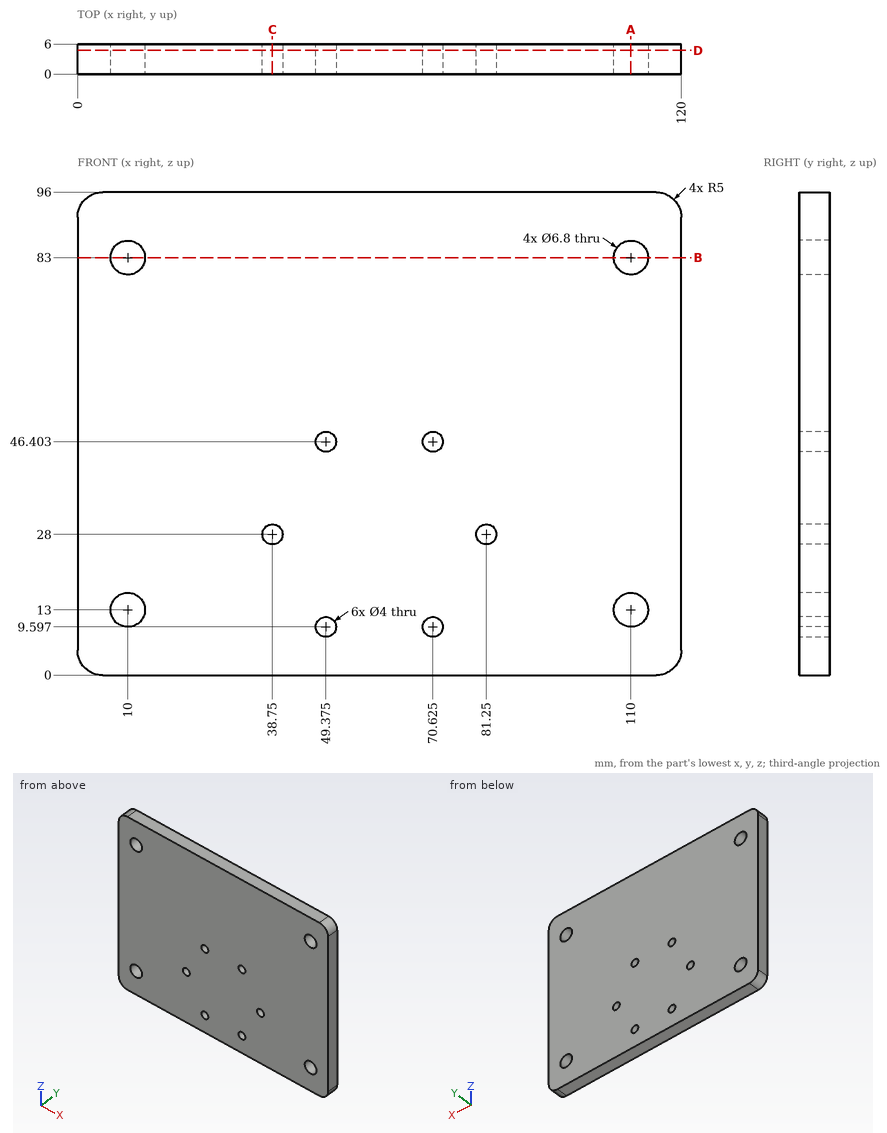
Part print with two shaded views. Sizes in mm from the minimum x, y, z corner. Round coordinates to 2 decimals unless told otherwise and drop trailing zeros. Loops run counter-clockwise (first coordinate to the right, second up) from the corner with the lowest first, then second, coordinate; pieces in that order, holes last. Notation, with made-up numbers: (40.5, -29) - (75.5, -29) arc R10 cw to (75.5, -23) - close; hole circle Ø3 at (47.5, 85.25). An arc over 180 degrees is marked (long way). Answer as a JSON object with one key per item and string values.
Item 1: Band-saw the part on A-A on x = 110. List the corners of the cut face in (y, z).
Output:
{"outline": "(0, 0) - (6, 0) - (6, 9.6) - (0, 9.6) - close; (0, 16.4) - (6, 16.4) - (6, 79.6) - (0, 79.6) - close; (0, 86.4) - (6, 86.4) - (6, 96) - (0, 96) - close"}
Item 2: Wall check: L1, parallel to Z at x = 10, y = 3; L2, parallel to Z at x = 49.5, y = 0.3; L3, parallel to Z at x = 81.5, y = 3.2. Give the ranges that are in metal, low to high.
Output:
{"L1": "0 to 9.6, 16.4 to 79.6, 86.4 to 96", "L2": "0 to 7.6, 11.59 to 44.41, 48.4 to 96", "L3": "0 to 26.02, 29.98 to 96"}
Item 3: Band-saw the part on B-B on z = 83. List the corners of the cut face in (x, y).
Output:
{"outline": "(0, 0) - (6.6, 0) - (6.6, 6) - (0, 6) - close; (13.4, 0) - (106.6, 0) - (106.6, 6) - (13.4, 6) - close; (113.4, 0) - (120, 0) - (120, 6) - (113.4, 6) - close"}
Item 4: Band-saw the part on D-D on y = 4.75. State how many separate pieces and enclosed holes the cut face has, plus the area to 3 significant figures.
Output:
{"separate pieces": "1", "enclosed holes": "10", "area": "11,300 mm2"}
Item 5: Band-saw the part on C-C on x = 38.75. List the corners of the cut face in (y, z), plus the area to 3 significant figures.
Output:
{"outline": "(0, 0) - (6, 0) - (6, 26) - (0, 26) - close; (0, 30) - (6, 30) - (6, 96) - (0, 96) - close", "area": "552 mm2"}
